Input: part model. Units: mm. Frame: model coordinates. A direction names the side the tool comes from. Give positions to 0.01 mm unless a question says otherwise; leave off trailing zeros. Order: outer loops, then holes, each group sorted by start corner. A loop starts at its lowest first (then second) coordinate and runs counter-clockwise, first axis right, second up. Notation, with made-up numbers: (75, 74) - (120, 74) arc R23 ccw to (120, 83) - close; hole circle Ø6 at (47, 31.25). An arc over 180 degrees is marked (long way). Answer in a Markdown table with one row per item. Add a question column.
1. Section query D-D on z = 160. Return loops of the section in (x, y), and give its area (3 significant figures).
2. Contact query for flat-ended pins moving along their axis: pin 1 (4 mm diameter, centred on x = 6, y = 3, fed in from -Z); pin 2 (8 mm diameter, centred on y = -1.5, z = 274, fed in from -X); pin 3 (1.5 mm diameter, centred on y = -6, z = 346, fed in from +X); pin 4 (6 mm diameter, centred on y = -1.5, z = 159, fed in from +X). Output: stop coordinate, or through.
3. Access query for faces 1 (the face through (-2.038, 9.176, 362.325)), 2 (the face through (2, -4, 350)). Directions: +Z, -Z, +X, -X, +Y, -Y. A direction counts if a zero-diameter tool reaches every point of the face in a straight line with its end or side. Return the directions, or none.
4. Section query C-C on z = 355. Return loops of the section in (x, y), and give its area (3 significant figures).
5. Ray query, line 1 (Z direction, x = -3.25, y = 4.5); line 2 (Y direction, x = -0.5, z = 194.5). Return the intervals inside material, ascending. Write a range as [from, to].
6. Section query A-A on y = 0. Return loops of the section in (x, z), and give its area (3 significant figures).
Autodesk Inventor part; units mm, degrees
ref_plane "YZ Plane" through (0, 0, 0) normal (1, 0, 0) x (0, 1, 0)
ref_plane "XZ Plane" through (0, 0, 0) normal (0, 1, 0) x (-1, 0, 0)
ref_plane "XY Plane" through (0, 0, 0) normal (0, 0, 1) x (1, 0, 0)
sketch "Sketch1" plane through (0, 0, 0) normal (0, 0, 1) x (1, 0, 0)
  circle A0 centre (0, 0) radius 4
  dimension "d0" = 8
extrude "Extrusion1" add sketch "Sketch1" along normal blind 350
sketch "Sketch2" plane through (0, 0, 350) normal (0, 0, 1) x (1, 0, 0)
  circle A0 centre (0, 0) radius 9.4
  dimension "d3" = 18.8
extrude "Extrusion2" add sketch "Sketch2" along normal blind 25
thread "Thread1"
sketch "Sketch3" plane through (0, 0, 0) normal (0, 0, -1) x (-1, 0, 0)
  circle A0 centre (0, 0) radius 4
extrude "Extrusion3" cut sketch "Sketch3" against normal blind 120
properties part number "00_spindel_350mm"
Answer:
| question | item | result |
|---|---|---|
| 1 | outline | circle Ø8 at (0, 0) |
| 1 | area | 50.3 mm² |
| 2 | pin 1 | stops at z = 350 |
| 2 | pin 2 | stops at x = -4 |
| 2 | pin 3 | passes through |
| 2 | pin 4 | stops at x = 4 |
| 3 | face 1 | +Z, -Z |
| 3 | face 2 | -Z |
| 4 | outline | circle Ø18.8 at (0, 0) |
| 4 | area | 278 mm² |
| 5 | line 1 | z = [350, 375] |
| 5 | line 2 | y = [-3.97, 3.97] |
| 6 | outline | (-9.4, 350) - (-4, 350) - (-4, 120) - (4, 120) - (4, 350) - (9.4, 350) - (9.4, 375) - (-9.4, 375) - close |
| 6 | area | 2,310 mm² |
